```python
from build123d import *

# Parameters (mm, degrees)
F0_W     = 19
F0_H     = 20.5
F0_W_2   = 5
F0_H_2   = 16.5
F0_W_3   = 10
F0_H_3   = 8.5
F0_W_4   = 2.5
F1_DEPTH = 3
F2_DEPTH = 6
F0_W_5   = 2
F0_H_4   = 10
F3_DEPTH = 7
F0_W_6   = 50
F0_H_5   = 2
F4_DEPTH = 12
F5_DEPTH = 1


with BuildPart() as f1:
    # F0 (on Top) → F1 (new body)
    with BuildSketch(Plane.XY):
        with Locations((61.5, 16.25)):
            Rectangle(F0_W, F0_H)
        Polygon((2, 6), (2, 2), (52, 2), (52, 6), (52, 26.5), (2, 26.5), (2, 22.5), (8, 22.5), (8, 6), align=None)
        with Locations((16.5, 14.25)):
            Rectangle(F0_W_2, F0_H_2, mode=Mode.SUBTRACT)
        with Locations((38.3, 14.25)):
            Rectangle(F0_W_3, F0_H_3, mode=Mode.SUBTRACT)
        with Locations((72.25, 16.25)):
            Rectangle(F0_W_4, F0_H)
    extrude(amount=F1_DEPTH)

    # F0 (on Top) → F2 (join)
    with BuildSketch(Plane.XY):
        Polygon((2, 19.25), (2, 9.25), (2, 6), (8, 6), (8, 22.5), (2, 22.5), align=None)
        with Locations((16.5, 14.25)):
            Rectangle(F0_W_2, F0_H_2)
        with Locations((38.3, 14.25)):
            Rectangle(F0_W_3, F0_H_3)
    extrude(amount=F2_DEPTH)

    # F0 (on Top) → F3 (join)
    with BuildSketch(Plane.XY):
        with Locations((1, 14.25)):
            Rectangle(F0_W_5, F0_H_4)
    extrude(amount=F3_DEPTH)

    # F0 (on Top) → F4 (join)
    with BuildSketch(Plane.XY):
        with Locations((27, 27.5)):
            Rectangle(F0_W_6, F0_H_5)
        Polygon((0, 28.5), (0, 19.25), (2, 19.25), (2, 22.5), (2, 26.5), (2, 28.5), align=None)
        Polygon((0, 9.25), (0, 0), (2, 0), (2, 2), (2, 6), (2, 9.25), align=None)
        with Locations((27, 1)):
            Rectangle(F0_W_6, F0_H_5)
    extrude(amount=F4_DEPTH)

    # F0 (on Top) → F5 (join)
    with BuildSketch(Plane.XY):
        Polygon((52, 28.5), (52, 26.5), (71, 26.5), (73.5, 26.5), (73.5, 28.5), align=None)
        Polygon((52, 2), (52, 0), (73.5, 0), (73.5, 6), (71, 6), (52, 6), align=None)
    extrude(amount=F5_DEPTH)


solid = f1.part
```
Design review of the part built by this model. Coordinates are the model's own, in mm. A direction names the side the tool comes from. Give positions to 0.01 mm unless a question says otherwise; leave off trailing zeros. Order: outer loops, then holes, each group sorted by start corner. A loop starts at its lowest first (then second) coordinate and runs counter-clockwise, first axis right, second up. Notation, with made-up numbers: (26.25, 30.25) -> (79.25, 30.25) arc R30 ccw to (79.25, 53.25) -> close; hole circle Ø2 at (28.5, 2). An arc over 180 degrees is marked (long way). Write item = value, one per line. Start each with the question number.
(1) We need section C-C on x = 7. Write out the cut boundary in (y, z).
(2) Mouldability with a two-part tool opening along Y and no side actions: class faces 1 (the face through (22, 1, 12)), 2 (the face through (5, 22.5, 4)), 3 (the face through (29, 28.5, 6)) as +Y half, -Y half, draft (parallel to the pull), parting line (faces both ways), or undercut.
(3) We need section D-D on y = 15.75. Write out the cut boundary in (x, z), plus the area to 4 significant figures.
(4) We need section B-B on z = 3.75. Write out the cut boundary in (x, y), plus the area to 4 significant figures.
(5) We need section A-A on z = 8.5. Write out the cut boundary in (x, y).
(6) For faces 4 (the face through (1, 19.25, 9)), 5 (the face through (16, 22.5, 4)), 6 (the face through (63, 6, 2)), list the 3-axis set-ups (+Z, -Z, +X, -X, +Y, -Y) from which the entire face can be reached by the end or side of a thin tool; tool diameter is ignored.
(7) To check wall thickness, follow line 1 along X through (y, z) = (14.75, 3.75); line 2 along Y through (x, z) = (19, 9.5); line 3 along X through (y, z) = (19, 4). State the ranges of each line that lie inside material, in increasing order.
(8) For pin 1 (1.8 mm diameter, centred on x = 57.5, y = 2.5, fed in from +Z); pin 2 (1.5 mm diameter, centred on x = 17.5, z = 5, fed in from -Y); pin 3 (1.8 mm diameter, centred on x = 4.5, y = 11.5, fed in from +Z); pin 4 (2 mm diameter, centred on y = 5.5, z = 8.5, fed in from +X), all flat-tipped, find the tip position at first contact; note any pin that passes through.
Numbers:
q1.outline = (0, 0) -> (28.5, 0) -> (28.5, 12) -> (26.5, 12) -> (26.5, 3) -> (22.5, 3) -> (22.5, 6) -> (6, 6) -> (6, 3) -> (2, 3) -> (2, 12) -> (0, 12) -> close
q2.face_1 = draft
q2.face_2 = undercut
q2.face_3 = +Y half
q3.outline = (0, 0) -> (73.5, 0) -> (73.5, 3) -> (43.3, 3) -> (43.3, 6) -> (33.3, 6) -> (33.3, 3) -> (19, 3) -> (19, 6) -> (14, 6) -> (14, 3) -> (8, 3) -> (8, 6) -> (2, 6) -> (2, 7) -> (0, 7) -> close
q3.area = 291.5 mm^2
q4.outline = (0, 0) -> (52, 0) -> (52, 2) -> (2, 2) -> (2, 6) -> (8, 6) -> (8, 22.5) -> (2, 22.5) -> (2, 26.5) -> (52, 26.5) -> (52, 28.5) -> (0, 28.5) -> close; (14, 6) -> (19, 6) -> (19, 22.5) -> (14, 22.5) -> close; (33.3, 10) -> (43.3, 10) -> (43.3, 18.5) -> (33.3, 18.5) -> close
q4.area = 523.5 mm^2
q5.outline = (0, 0) -> (52, 0) -> (52, 2) -> (2, 2) -> (2, 9.25) -> (0, 9.25) -> close; (0, 19.25) -> (2, 19.25) -> (2, 26.5) -> (52, 26.5) -> (52, 28.5) -> (0, 28.5) -> close
q6.face_4 = +Z, +X, -X
q6.face_5 = +Z, +X
q6.face_6 = +Z, +X, -Y
q7.line_1 = 0 to 8, 14 to 19, 33.3 to 43.3
q7.line_2 = 0 to 2, 26.5 to 28.5
q7.line_3 = 0 to 8, 14 to 19
q8.pin_1 = 1
q8.pin_2 = 0
q8.pin_3 = 6
q8.pin_4 = 2
